Design review of the part built by this model. Coordinates are the model's own, in mm. Face numbers are marked on the shaded views. A direction names the side the tool comes from. Round coordinates to 2 decimals unless told otherwise and drop trailing zeros. Order: outer loops, then holes, each group sorted by start corner. A loop starts at its lowest first (then second) coordinate and runs counter-clockwise, first axis right, second up. Notation, with made-up numbers: (59.25, 75) - (111.25, 75) arc R30 cw to (111.25, 100) - close; hole circle Ø1 at (-23.5, 50). An arc over 180 degrees is marked (long way). Use CSV: the item, a comma, the result in double quotes.
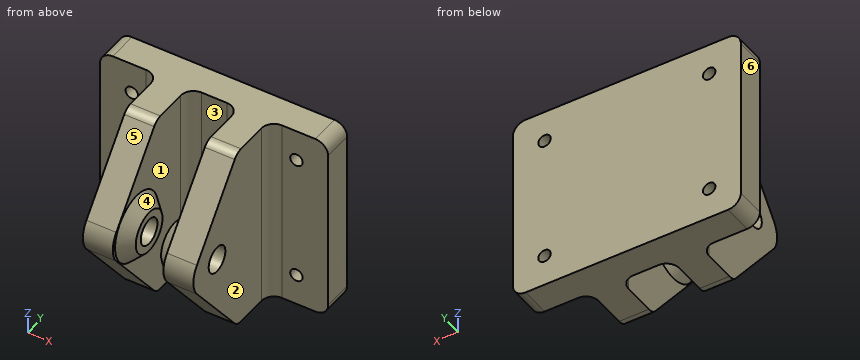
from build123d import *
from OCP.BRepFilletAPI import BRepFilletAPI_MakeFillet

# Parameters (mm, degrees)
SKETCH1_R           = 2.627
BOSS_EXTRUDE1_DEPTH = 6
BOSS_EXTRUDE2_START = -5.08
SKETCH1_3_W         = 38.1
SKETCH1_3_H         = 5.999999938
BOSS_EXTRUDE2_DEPTH = 22.86
SKETCH3_R           = 1.25
CUT_EXTRUDE1_DEPTH  = 44.260167546
FILLET1_R1          = 2.54
FILLET1_R2          = 5.08
SKETCH4_R           = 4.2145
SKETCH4_R_2         = 2.627
BOSS_EXTRUDE3_DEPTH = 2.54
BOSS_EXTRUDE4_START = 7.62
SKETCH4_2_R         = 4.2145
SKETCH4_2_R_2       = 2.627
BOSS_EXTRUDE4_DEPTH = 2.54
CHAMFER2_SIZE       = 2.54


with BuildPart() as part:
    # Sketch1 → Boss-Extrude1 (new body)
    with BuildSketch(Plane(origin=(5.08, 0, 0), x_dir=(0, 0, -1), z_dir=(1, 0, 0))):
        Polygon((-19.05, 0), (-19.05, -10.16), (0, -25.4), (19.05, -10.16), (19.05, 0), align=None)
        with Locations((0, -16.51)):
            Circle(SKETCH1_R, mode=Mode.SUBTRACT)
    boss_extrude1 = extrude(amount=BOSS_EXTRUDE1_DEPTH)

    # Sketch1<3> → Boss-Extrude2 (add)
    with BuildSketch(Plane(origin=(5.08, 0, 0), x_dir=(0, 0, -1), z_dir=(1, 0, 0)).offset(BOSS_EXTRUDE2_START)):
        with Locations((0, 2.999999969)):
            Rectangle(SKETCH1_3_W, SKETCH1_3_H)
    boss_extrude2 = extrude(amount=BOSS_EXTRUDE2_DEPTH)

    # Sketch3 → Cut-Extrude1 (cut, through all)
    with BuildSketch(Plane(origin=(0, 5.999999938, 0), x_dir=(1, 0, 0), z_dir=(0, 1, 0))):
        with Locations(Location((16.51, 12.7, 0), (0, 0, 270))):
            Circle(SKETCH3_R)
        with Locations(Location((16.51, -12.7, 0), (0, 0, 90))):
            Circle(SKETCH3_R)
    cut_extrude1 = extrude(amount=-CUT_EXTRUDE1_DEPTH, mode=Mode.SUBTRACT)

    # Mirror2: Boss-Extrude2, Cut-Extrude1 across plane
    add(boss_extrude2.mirror(Plane(origin=(0, 0, 0), x_dir=(0, 0, 1), z_dir=(1, 0, 0))))
    add(cut_extrude1.mirror(Plane(origin=(0, 0, 0), x_dir=(0, 0, 1), z_dir=(1, 0, 0))), mode=Mode.SUBTRACT)

    # Mirror3: Boss-Extrude1 across plane
    add(boss_extrude1.mirror(Plane(origin=(0, 0, 0), x_dir=(0, 0, 1), z_dir=(1, 0, 0))))

    # Fillet1: one fillet with a radius per group of edges: ONE call of the kernel's fillet builder (fillet() takes one radius for all edges)
    fillet1_edges_1 = [part.edges().sort_by_distance(p)[0] for p in [
        (8.08, -10.16, 19.05),
        (8.08, -10.16, -19.05),
        (11.08, 0, 0),
        (22.86, 2.999999969, 19.05),
        (22.86, 2.999999969, -19.05),
        (-22.86, 2.999999969, -19.05),
        (-22.86, 2.999999969, 19.05),
        (-8.08, -10.16, -19.05),
        (-8.08, -10.16, 19.05),
        (-5.08, 0, 0),
        (-11.08, 0, 0),
        (5.08, 0, 0),
    ]]
    fillet1_edges_2 = [part.edges().sort_by_distance(p)[0] for p in [
        (8.08, -25.4, 0),
        (-8.08, -25.4, 0),
    ]]
    fillet1 = BRepFilletAPI_MakeFillet(part.part.solid().wrapped)
    for e in fillet1_edges_1:
        fillet1.Add(FILLET1_R1, e.wrapped)
    for e in fillet1_edges_2:
        fillet1.Add(FILLET1_R2, e.wrapped)
    add(Compound.cast(fillet1.Shape()), mode=Mode.REPLACE)

    # Sketch4 → Boss-Extrude3 (add)
    with BuildSketch(Plane.ZY.offset(-5.08)):
        with Locations(Location((0, -16.51, 0), (0, 0, 180))):
            Circle(SKETCH4_R)
        with Locations((0, -16.51)):
            Circle(SKETCH4_R_2, mode=Mode.SUBTRACT)
    extrude(amount=BOSS_EXTRUDE3_DEPTH)

    # Sketch4<2> → Boss-Extrude4 (add)
    with BuildSketch(Plane.ZY.offset(-5.08).offset(BOSS_EXTRUDE4_START)):
        with Locations(Location((0, -16.51, 0), (0, 0, 180))):
            Circle(SKETCH4_2_R)
        with Locations((0, -16.51)):
            Circle(SKETCH4_2_R_2, mode=Mode.SUBTRACT)
    extrude(amount=BOSS_EXTRUDE4_DEPTH)

    # Chamfer2
    chamfer2_edges = [part.edges().sort_by_distance(p)[0] for p in [
        (5.08, -16.51, 4.2145),
        (-5.08, -16.51, 4.2145),
    ]]
    chamfer(chamfer2_edges, length=CHAMFER2_SIZE - 0.0001)  # a hair under: the kernel refuses the full size


solid = part.part
1) For the marked faces 1, 2 and 3, list the 3-axis set-ups (+Z, -Z, +X, -X, +Y, -Y) from which the entire face can be reached by the end or side of a thin tool; tool diameter is ignored.
Data:
face 1,"none"
face 2,"+Z, -Z, +X, -Y"
face 3,"+Z, -Z, -Y"
2) We need section A-A (y = -6.5). Give the boundary of the cut face in (x, z).
Data:
outline,"(-11.08, -19.05) - (-5.08, -19.05) - (-5.08, 19.05) - (-11.08, 19.05) - close; (5.08, -19.05) - (11.08, -19.05) - (11.08, 19.05) - (5.08, 19.05) - close"
3) The part is to be moulded in two halves that separate along Y. For the marked faces 4, 5 and 6, say which applies: +Y half, -Y half, draft (parallel to the pull), parting line (faces both ways), or undercut.
Data:
face 4,"undercut"
face 5,"-Y half"
face 6,"draft"
4) Insertion check: pin 1 Ø4 at (y, z) = (-16.51, 0) entering from -X; pin 2 Ø5 at (x, z) = (-2, 4.5) entering from -Y; pin 3 Ø10 at (y, z) = (-17.5, 11.5) entering from +X; pin 4 Ø3 at (x, z) = (-16.51, 12.7) entering from +Y. Each pin has a flat end and moves straight along its axis. Give the tip position at first contact, or say it passes through.
Data:
pin 1,"passes through"
pin 2,"stops at y = -21.36"
pin 3,"stops at x = 11.08"
pin 4,"stops at y = 6"
5) To check wall thickness, follow L1, parallel to X at y = 2.55, z = 12.7; L2, parallel to Y at x = -9.4, z = 0; L3, parallel to Y at x = -4.05, z = 0. State the ranges of each line that lie inside material, in increasing order. Write a range as from..to.
Data:
L1,"x = -22.86..-17.76, -15.26..15.26, 17.76..22.86"
L2,"y = -23.97..-19.14, -13.88..6"
L3,"y = -22.23..-19.14, -13.88..-10.79, -0.5..6"
6) We need section C-C (z = 12.7). Give the boundary of the cut face in (x, y).
Data:
outline,"(-22.86, 0) - (-17.76, 0) - (-17.76, 6) - (-22.86, 6) - close; (-15.26, 0) - (-13.62, 0) arc R2.54 cw to (-11.08, -2.54) - (-11.08, -15.24) - (-5.08, -15.24) - (-5.08, -2.54) arc R2.54 cw to (-2.54, 0) - (2.54, 0) arc R2.54 cw to (5.08, -2.54) - (5.08, -15.24) - (11.08, -15.24) - (11.08, -2.54) arc R2.54 cw to (13.62, 0) - (15.26, 0) - (15.26, 6) - (-15.26, 6) - close; (17.76, 0) - (22.86, 0) - (22.86, 6) - (17.76, 6) - close"
7) We need section B-B (x = 16.51). Give the boundary of the cut face in (y, z), then the cut area to 3 significant figures.
Data:
outline,"(0, -19.05) - (6, -19.05) - (6, -13.95) - (0, -13.95) - close; (0, -11.45) - (6, -11.45) - (6, 11.45) - (0, 11.45) - close; (0, 13.95) - (6, 13.95) - (6, 19.05) - (0, 19.05) - close"
area,"199 mm2"
8) We need section D-D (z = 8.5). Give the boundary of the cut face in (x, y), then the cut area to 3 significant figures.
Data:
outline,"(-22.86, 0) - (-13.62, 0) arc R2.54 cw to (-11.08, -2.54) - (-11.08, -18.6) - (-5.08, -18.6) - (-5.08, -2.54) arc R2.54 cw to (-2.54, 0) - (2.54, 0) arc R2.54 cw to (5.08, -2.54) - (5.08, -18.6) - (11.08, -18.6) - (11.08, -2.54) arc R2.54 cw to (13.62, 0) - (22.86, 0) - (22.86, 6) - (-22.86, 6) - close"
area,"503 mm2"
